```python
from build123d import *

# Parameters (mm, degrees)
SKETCH7_R                = 16
BOSS_EXTRUDE3_DEPTH      = 10
SKETCH8_R                = 7.25
CUT_EXTRUDE8_DEPTH       = 10
SKETCH9_R                = 14
SKETCH9_R_2              = 7.75
CUT_EXTRUDE9_DEPTH       = 8
BOSS_EXTRUDE5_DEPTH      = 8
BOSS_EXTRUDE5_DEPTH_BACK = 2
CUT_EXTRUDE11_DEPTH      = 8
BOSS_EXTRUDE6_DEPTH      = 10


with BuildPart() as part:
    # Sketch7 → Boss-Extrude3 (new body)
    with BuildSketch(Plane(origin=(0, 0, 0), x_dir=(1, 0, 0), z_dir=(0, 1, 0))):
        with Locations(Location((0, 0, 0), (0, 0, 270))):
            Circle(SKETCH7_R)
    extrude(amount=BOSS_EXTRUDE3_DEPTH)

    # Sketch8 → Cut-Extrude8 (cut)
    with BuildSketch(Plane(origin=(0, 0, 0), x_dir=(1, 0, 0), z_dir=(0, 1, 0))):
        with Locations(Location((0, 0, 0), (0, 0, 270))):
            Circle(SKETCH8_R)
    extrude(amount=CUT_EXTRUDE8_DEPTH, mode=Mode.SUBTRACT)

    # Sketch9 → Cut-Extrude9 (cut)
    with BuildSketch(Plane(origin=(0, 10, 0), x_dir=(1, 0, 0), z_dir=(0, 1, 0))):
        with Locations(Location((0, 0, 0), (0, 0, 270))):
            Circle(SKETCH9_R)
        with Locations(Location((0, 0, 0), (0, 0, 270))):
            Circle(SKETCH9_R_2, mode=Mode.SUBTRACT)
    extrude(amount=-CUT_EXTRUDE9_DEPTH, mode=Mode.SUBTRACT)

    # Sketch10 → Boss-Extrude5 (add, two sides: drawn at the far end of the back side and taken through both)
    with BuildSketch(Plane(origin=(0, 2, 0), x_dir=(1, 0, 0), z_dir=(0, 1, 0)).offset(-BOSS_EXTRUDE5_DEPTH_BACK)):
        with BuildLine():
            Line((16, 0), (61, 0))
            Line((61, 0), (61, -120))
            Line((61, -120), (-61, -120))
            Line((-61, -120), (-61, 0))
            Line((-61, 0), (-16, 0))
            ThreePointArc((-16, 0), (0, -16), (16, 0))
        make_face()
    extrude(amount=BOSS_EXTRUDE5_DEPTH + BOSS_EXTRUDE5_DEPTH_BACK)

    # Sketch11 → Cut-Extrude11 (cut)
    with BuildSketch(Plane(origin=(0, 10, 0), x_dir=(1, 0, 0), z_dir=(0, 1, 0))):
        with BuildLine():
            Line((-59, -2), (-59, -118))
            Line((-59, -118), (59, -118))
            Line((59, -118), (59, -2))
            Line((59, -2), (13.856406461, -2))
            ThreePointArc((13.856406461, -2), (0, -14), (-13.856406461, -2))
            Line((-13.856406461, -2), (-59, -2))
        make_face()
    extrude(amount=-CUT_EXTRUDE11_DEPTH, mode=Mode.SUBTRACT)

    # Sketch12 → Boss-Extrude6 (add)
    with BuildSketch(Plane(origin=(0, 2, 0), x_dir=(1, 0, 0), z_dir=(0, 1, 0))):
        Polygon((-59, -118), (-61, -118), (-61, -120), (61, -120), (61, -118), align=None)
    extrude(amount=BOSS_EXTRUDE6_DEPTH)


solid = part.part
```
Verification items for the finished model (mm, model axes). A direction names the side the tool comes from. Round coordinates to 2 decimals unless told otherwise and drop trailing zeros. Order: outer loops, then holes, each group sorted by start corner. A loop starts at its lowest first (then second) coordinate and runs counter-clockwise, first axis right, second up. Notation, with made-up numbers: (27, 19.25) -> (31, 19.25) arc R17 cw to (31, 47.25) -> close; hole circle Ø3 at (-2.75, 29). An arc over 180 degrees is marked (long way). Put each result on its own line as item: value. Start each with the question number.
(1) Tool access check on faces 1 (the face through (-39, 5, 0)), 2 (the face through (61, 5, 59)), 3 (the face through (37, 6, 2)), 4 (the face through (27, 10, 1)). Record the directions out of +Z, -Z, +X, -X, +Y, -Y that give a thin tool (end or side, any length) a straight path to the whole face; none if there is none.
(2) Section check A-A (y = 7.25). Enter the section's corners in (x, z), then the cut area to 3 significant figures.
(3) Depth check by flat-ended pin: pin 1 Ø8.5 at (x, z) = (0, 0) entering from -Y; pin 2 Ø1 at (x, z) = (-15, 98) entering from +Y; pin 3 Ø3 at (x, y) = (29.5, 5) entering from -Z; pin 4 Ø25 at (x, z) = (0, 0) entering from +Y. Enter the tip coordinate at first touch or a pass-through.
(4) Material ranges on line 1 along X through (y, z) = (7, 40); line 2 along Z through (x, y) = (39, 5); line 3 along Z through (x, y) = (4, 5.5), recorded low to high.
(5) Section check D-D (x = 19.5). Enter the section's corners in (y, z), then the cut area to 3 significant figures.
(6) Draft check along Z on faces 5 (the face through (-2.8, 10, 6.9)), 6 (the face through (0, 6, -14)), 7 (the face through (38, 5, 0)). Enter one of: +Z half, -Z half, draft (parallel to the pull), parting line (faces both ways), or undercut.
(7) Section check B-B (x = 0). Enter the section's corners in (y, z).
(8) Section check C-C (z = -5.5). Enter the section's corners in (x, y), then the cut area to 3 significant figures.
Completed:
1. face 1: -Z, -X, +Y, -Y
1. face 2: +Z, -Z, +X, +Y, -Y
1. face 3: +Y
1. face 4: -Z, +X, -X, +Y
2. outline: (-61, 0) -> (-16, 0) arc R16 ccw to (16, 0) -> (61, 0) -> (61, 120) -> (-61, 120) -> close; circle Ø15.5 at (0, 0); hole (-59, 2) -> (-13.86, 2) arc R14 ccw (long way) to (13.86, 2) -> (59, 2) -> (59, 118) -> (-59, 118) -> close; hole circle Ø14.5 at (0, 0)
2. area: 1,010 mm2
3. pin 1: passes through
3. pin 2: stops at y = 2
3. pin 3: stops at z = 0
3. pin 4: stops at y = 10
4. line 1: x = -61 to -59, 59 to 61
4. line 2: z = 0 to 2, 118 to 120
4. line 3: z = -15.49 to -13.42, -6.64 to -6.05, 6.05 to 6.64, 118 to 120
5. outline: (0, 0) -> (10, 0) -> (10, 2) -> (2, 2) -> (2, 118) -> (12, 118) -> (12, 120) -> (0, 120) -> close
5. area: 276 mm2
6. face 5: draft
6. face 6: undercut
6. face 7: -Z half
7. outline: (0, -16) -> (10, -16) -> (10, -14) -> (2, -14) -> (2, -7.75) -> (10, -7.75) -> (10, -7.25) -> (0, -7.25) -> close; (0, 7.25) -> (10, 7.25) -> (10, 7.75) -> (2, 7.75) -> (2, 118) -> (12, 118) -> (12, 120) -> (0, 120) -> close
8. outline: (-15.02, 0) -> (-4.72, 0) -> (-4.72, 10) -> (-5.46, 10) -> (-5.46, 2) -> (-12.87, 2) -> (-12.87, 10) -> (-15.02, 10) -> close; (4.72, 0) -> (15.02, 0) -> (15.02, 10) -> (12.87, 10) -> (12.87, 2) -> (5.46, 2) -> (5.46, 10) -> (4.72, 10) -> close
8. area: 87.4 mm2
